Geometry check sheet. Reference: drawing and pictorial views, mm from the part's lowest x, y, z. A direction names the side the tool comes from. Round coordinates to 2 decimals unless told otherwise and drop trailing zeros. Loops run counter-clockwise (first coordinate to the right, second up) from the corner with the lowest first, then second, coordinate; pieces in that order, holes last. Notation, with made-up numbers: (-13, 19) - (7, 19) arc R22 cw to (7, 41) - close; hole circle Ø3 at (-15, -10). An arc over 180 degrees is marked (long way). Put each result on its own line as item: value. Start each with the question number.
Item 1: Draft check along Y on the marked faces 1, 2, 3 and 4. Enter one of: pulls with the +Y half, pulls with the -Y half, needs draft (parallel to the pull), parting line crosses it, or undercut.
Item 2: Section check A-A, the plane x = 17.25. Record the cut outline in (y, z).
Item 3: Section check C-C, the plane y = 35. Record the cut outline in (x, z).
Item 4: Section check D-D, the plane x = 23. Record the cut outline in (y, z).
Item 5: Section check B-B, the plane z = 2.25. Record the cut outline in (x, y).
Item 6: Material ranges on line 1 along Y through (x, z) = (25.5, 4.5); line 2 along Z through (x, y) = (2, 22.5); line 3 along X through (y, z) = (8, 3.75), recorded low to high.
Item 7: Tool access check on the marked faces 5 and 6. Record the directions out of +Z, -Z, +X, -X, +Y, -Y that give a thin tool (end or side, any length) a straight path to the whole face; none if there is none.
Item 8: Gauge pin test, flat ends, axial feed: pin 1 Ø2 at (y, z) = (29.5, 2.5) entering from +X; pin 2 Ø1.5 at (y, z) = (10, 1) entering from -X; pin 3 Ø2.5 at (y, z) = (41, 6) entering from +X. Record the tip position at first contact, or that the pin passes through.
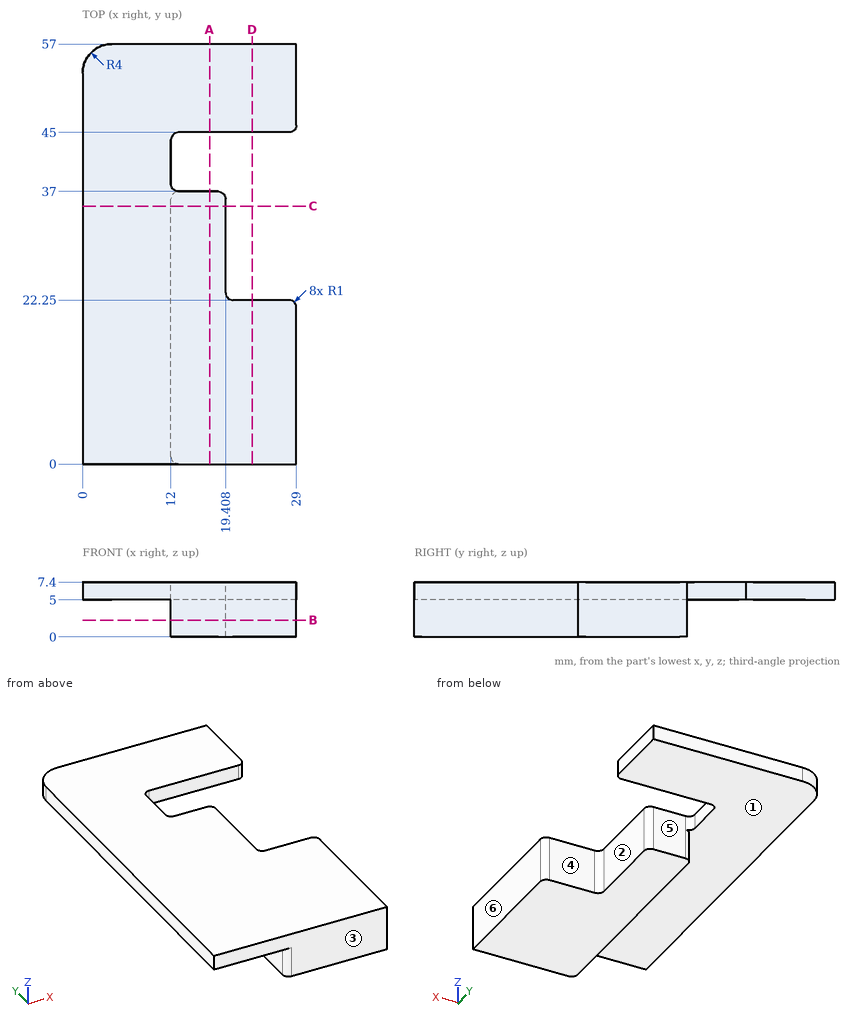
Check result:
1. face 1: needs draft
1. face 2: undercut
1. face 3: pulls with the -Y half
1. face 4: undercut
2. outline: (0, 0) - (37, 0) - (37, 7.4) - (0, 7.4) - close; (45, 5) - (57, 5) - (57, 7.4) - (45, 7.4) - close
3. outline: (0, 5) - (12, 5) - (12, 0) - (19.41, 0) - (19.41, 7.4) - (0, 7.4) - close
4. outline: (0, 0) - (22.25, 0) - (22.25, 7.4) - (0, 7.4) - close; (45, 5) - (57, 5) - (57, 7.4) - (45, 7.4) - close
5. outline: (12, 1) arc R1 ccw to (13, 0) - (29, 0) - (29, 21.25) arc R1 ccw to (28, 22.25) - (20.41, 22.25) arc R1 cw to (19.41, 23.25) - (19.41, 36) arc R1 ccw to (18.41, 37) - (13, 37) arc R1 ccw to (12, 36) - close
6. line 1: 0 to 22.25
6. line 2: 5 to 7.4
6. line 3: 12 to 29
7. face 5: +Z, -Z, +X
7. face 6: +Z, -Z, +X, +Y, -Y
8. pin 1: x = 19.41
8. pin 2: x = 12
8. pin 3: x = 12
